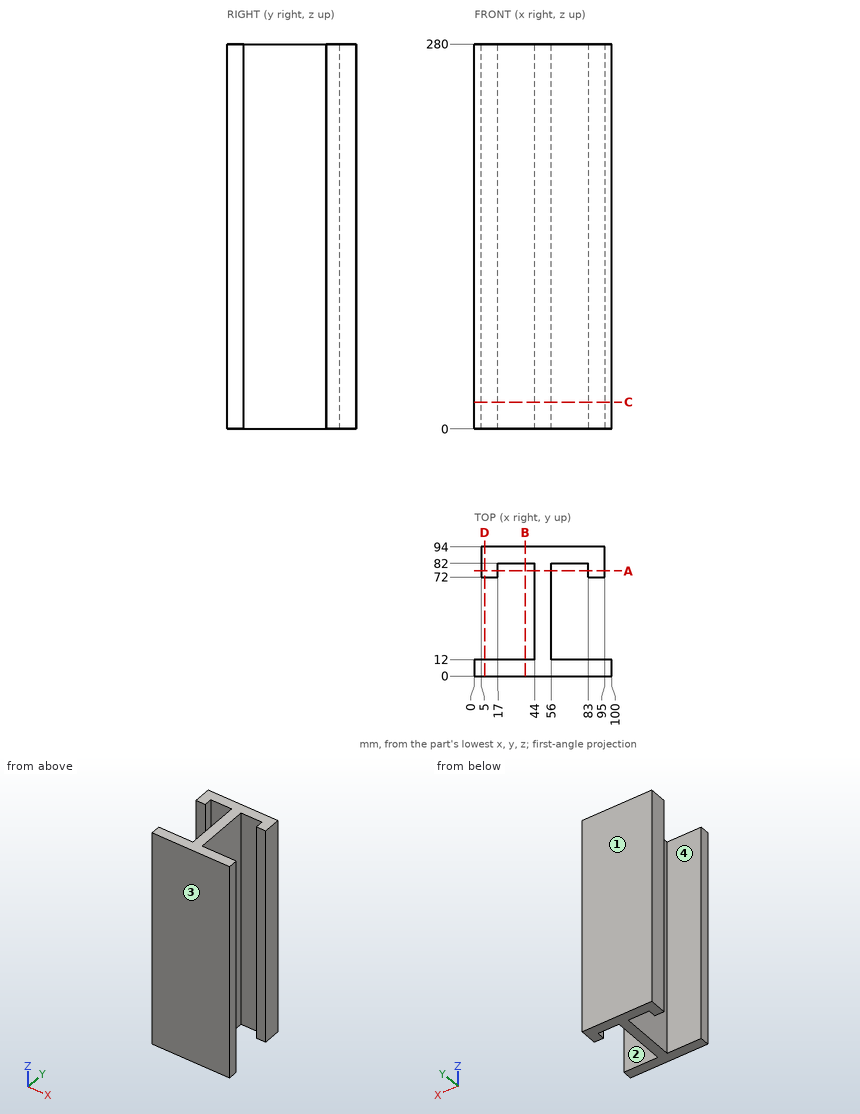
For this review, use the dimensioned drawing (mm, ordinates from the lowest corner) and the shaded views. Give positions to 0.01 mm unless a question says otherwise; leave off trailing zeros. Order: outer loops, then holes, each group sorted by start corner. A loop starts at its lowest first (then second) coordinate and runs counter-clockwise, first axis right, second up.
1. Add section B-B, the plane x = 37. State the section outline as (y, z) points, then the cut area to 3 significant figures.
Solution:
outline: (0, 0) - (12, 0) - (12, 280) - (0, 280) - close; (82, 0) - (94, 0) - (94, 280) - (82, 280) - close
area: 6,720 mm2
2. Mouldability with a two-part tool opening along Y and no side actions: class the marked faces 1, 2, 3 and 4 as +Y half, -Y half, draft (parallel to the pull), parting line (faces both ways), or undercut.
Solution:
face 1: +Y half
face 2: undercut
face 3: -Y half
face 4: undercut
3. For pin 1 Ø21 at (y, z) = (46.5, 187) entering from -X; pin 2 Ø21 at (y, z) = (45, 135.5) entering from +X; pin 3 Ø8 at (y, z) = (75.5, 127) entering from -X, all flat-tipped, find the tip position at first contact; note any pin that passes through.
Solution:
pin 1: stops at x = 44
pin 2: stops at x = 56
pin 3: stops at x = 5
4. To check wall thickness, follow L1, parallel to Y at x = 27.5, z = 17; L2, parallel to Y at x = 14, z = 156; L3, parallel to X at y = 23.5, z = 221. State the ranges of each line that lie inside material, in increasing order.
Solution:
L1: y = 0 to 12, 82 to 94
L2: y = 0 to 12, 72 to 94
L3: x = 44 to 56
5. Add section A-A, the plane y = 76.5. State the section outline as (x, z) points.
Solution:
outline: (5, 0) - (17, 0) - (17, 280) - (5, 280) - close; (44, 0) - (56, 0) - (56, 280) - (44, 280) - close; (83, 0) - (95, 0) - (95, 280) - (83, 280) - close
6. Add section D-D, the plane x = 7.5. State the section outline as (y, z) points.
Solution:
outline: (0, 0) - (12, 0) - (12, 280) - (0, 280) - close; (72, 0) - (94, 0) - (94, 280) - (72, 280) - close
7. Add section C-C, the plane z = 19.5. State the section outline as (x, y) points, then the cut area to 3 significant figures.
Solution:
outline: (0, 0) - (100, 0) - (100, 12) - (56, 12) - (56, 82) - (83, 82) - (83, 72) - (95, 72) - (95, 94) - (5, 94) - (5, 72) - (17, 72) - (17, 82) - (44, 82) - (44, 12) - (0, 12) - close
area: 3,360 mm2
